Autodesk Fusion 360 part; units mm, degrees
sketch "スケッチ1" plane through (0, 0, 0) normal (0, 0, 1) x (1, 0, 0)
  line L0 (0, 0) -> (74, 0)
  line L1 (74, 0) -> (74, 46)
  line L2 (74, 46) -> (0, 46)
  line L3 (0, 46) -> (0, 0)
  dimension "d1" = 46
  dimension "d2" = 74
extrude "押し出し1" add sketch "スケッチ1" along normal blind 2
sketch "スケッチ2" plane through (0, 0, 2) normal (0, 0, 1) x (-1, 0, 0)
  line L0 (0, -46) -> (0, 0)
  line L1 (0, 0) -> (-74, 0)
  line L2 (-74, 0) -> (-74, -46)
  line L3 (-74, -46) -> (0, -46)
  line L4 (-27, -13) -> (-47, -13)
  line L5 (-47, -13) -> (-47, -15)
  line L6 (-47, -15) -> (-27, -15)
  line L7 (-27, -15) -> (-27, -13)
  dimension "d5" = 2
  dimension "d6" = 20
  dimension "d7" = 13
  dimension "d8" = 27
extrude "押し出し2" cut sketch "スケッチ2" against normal blind 2 contours L4 L5 L6 L7
sketch "スケッチ3" plane through (0, 0, 2) normal (0, 0, 1) x (-1, 0, 0)
  line L0 (-47, -13) -> (-27, -13)
  line L1 (-27, -13) -> (-27, -15)
  line L2 (-27, -15) -> (-47, -15)
  line L3 (-47, -15) -> (-47, -13)
  line L4 (0, -46) -> (0, 0)
  line L5 (0, 0) -> (-74, 0)
  line L6 (-74, 0) -> (-74, -46)
  line L7 (-74, -46) -> (0, -46)
  line L8 (-67, -46) -> (-58, -46)
  line L9 (-58, -46) -> (-58, -44)
  line L10 (-58, -44) -> (-67, -44)
  line L11 (-67, -44) -> (-67, -46)
  line L12 (-50, -46) -> (-41, -46)
  line L13 (-50, -44) -> (-50, -46)
  line L14 (-41, -44) -> (-50, -44)
  line L15 (-41, -46) -> (-41, -44)
  line L16 (-33, -46) -> (-24, -46)
  line L17 (-33, -44) -> (-33, -46)
  line L18 (-24, -44) -> (-33, -44)
  line L19 (-24, -46) -> (-24, -44)
  line L20 (-16, -46) -> (-7, -46)
  line L21 (-16, -44) -> (-16, -46)
  line L22 (-7, -44) -> (-16, -44)
  line L23 (-7, -46) -> (-7, -44)
  line L24 (-24, 0) -> (-33, 0)
  line L25 (-33, 0) -> (-33, -2)
  line L26 (-58, 0) -> (-67, 0)
  line L27 (-50, 0) -> (-50, -2)
  line L28 (-50, -2) -> (-41, -2)
  line L29 (-7, -2) -> (-7, 0)
  line L30 (-7, 0) -> (-16, 0)
  line L31 (-16, 0) -> (-16, -2)
  line L32 (-33, -2) -> (-24, -2)
  line L33 (-67, 0) -> (-67, -2)
  line L34 (-41, -2) -> (-41, 0)
  line L35 (-16, -2) -> (-7, -2)
  line L36 (-24, -2) -> (-24, 0)
  line L37 (-41, 0) -> (-50, 0)
  line L38 (-67, -2) -> (-58, -2)
  line L39 (-58, -2) -> (-58, 0)
  line L40 (0, -38) -> (-2, -38)
  line L41 (-2, -38) -> (-2, -32)
  line L42 (-2, -32) -> (0, -32)
  line L43 (0, -32) -> (0, -38)
  line L44 (-2, -20) -> (0, -20)
  line L45 (-2, -26) -> (-2, -20)
  line L46 (0, -26) -> (-2, -26)
  line L47 (0, -20) -> (0, -26)
  line L48 (-2, -8) -> (0, -8)
  line L49 (-2, -14) -> (-2, -8)
  line L50 (0, -14) -> (-2, -14)
  line L51 (0, -8) -> (0, -14)
  line L52 (-74, -20) -> (-72, -20)
  line L53 (-72, -8) -> (-72, -14)
  line L54 (-74, -8) -> (-72, -8)
  line L55 (-72, -14) -> (-74, -14)
  line L56 (-74, -38) -> (-74, -32)
  line L57 (-72, -32) -> (-72, -38)
  line L58 (-72, -26) -> (-74, -26)
  line L59 (-74, -32) -> (-72, -32)
  line L60 (-74, -14) -> (-74, -8)
  line L61 (-72, -20) -> (-72, -26)
  line L62 (-74, -26) -> (-74, -20)
  line L63 (-72, -38) -> (-74, -38)
  dimension "d11" = 9
  dimension "d12" = 2
  dimension "d13" = 7
  dimension "d16" = 17
  dimension "d17" = 0
  dimension "d20" = 0
  dimension "d21" = 44
  dimension "d22" = 6
  dimension "d23" = 2
  dimension "d24" = 8
  dimension "d27" = 0
  dimension "d28" = 12
  dimension "d31" = -72
  dimension "d32" = 0
extrude "押し出し3" cut sketch "スケッチ3" against normal blind 2 contours L4 L40 L41 L42 L43 | L7 L20 L21 L22 L23 | L4 L44 L45 L46 L47 | L7 L16 L17 L18 L19 | L4 L48 L49 L50 L51 | L7 L12 L13 L14 L15 | L7 L8 L9 L10 L11 | L5 L29 L30 L31 L35 | L5 L24 L25 L32 L36 | L6 L56 L57 L59 L63 | L5 L27 L28 L34 L37 | L6 L52 L58 L61 L62 | L5 L26 L33 L38 L39 | L6 L53 L54 L55 L60
sketch "スケッチ4" plane through (0, 0, 2) normal (0, 0, 1) x (-1, 0, 0)
  line L0 (-50, -2) -> (-50, 0)
  line L1 (-50, 0) -> (-58, 0)
  line L2 (-58, 0) -> (-58, -2)
  line L3 (-58, -2) -> (-67, -2)
  line L4 (-67, -2) -> (-67, 0)
  line L5 (-67, 0) -> (-74, 0)
  line L6 (-74, 0) -> (-74, -8)
  line L7 (-74, -8) -> (-72, -8)
  line L8 (-72, -8) -> (-72, -14)
  line L9 (-72, -14) -> (-74, -14)
  line L10 (-74, -14) -> (-74, -20)
  line L11 (-74, -20) -> (-72, -20)
  line L12 (-72, -20) -> (-72, -26)
  line L13 (-72, -26) -> (-74, -26)
  line L14 (-74, -26) -> (-74, -32)
  line L15 (-74, -32) -> (-72, -32)
  line L16 (-72, -32) -> (-72, -38)
  line L17 (-72, -38) -> (-74, -38)
  line L18 (-74, -38) -> (-74, -46)
  line L19 (-74, -46) -> (-67, -46)
  line L20 (-67, -46) -> (-67, -44)
  line L21 (-67, -44) -> (-58, -44)
  line L22 (-58, -44) -> (-58, -46)
  line L23 (-58, -46) -> (-50, -46)
  line L24 (-50, -46) -> (-50, -44)
  line L25 (-50, -44) -> (-41, -44)
  line L26 (-41, -44) -> (-41, -46)
  line L27 (-41, -46) -> (-33, -46)
  line L28 (-33, -46) -> (-33, -44)
  line L29 (-33, -44) -> (-24, -44)
  line L30 (-24, -44) -> (-24, -46)
  line L31 (-24, -46) -> (-16, -46)
  line L32 (-16, -46) -> (-16, -44)
  line L33 (-16, -44) -> (-7, -44)
  line L34 (-7, -44) -> (-7, -46)
  line L35 (-7, -46) -> (0, -46)
  line L36 (0, -46) -> (0, -38)
  line L37 (0, -38) -> (-2, -38)
  line L38 (-2, -38) -> (-2, -32)
  line L39 (-2, -32) -> (0, -32)
  line L40 (0, -32) -> (0, -26)
  line L41 (0, -26) -> (-2, -26)
  line L42 (-2, -26) -> (-2, -20)
  line L43 (-2, -20) -> (0, -20)
  line L44 (0, -20) -> (0, -14)
  line L45 (0, -14) -> (-2, -14)
  line L46 (-2, -14) -> (-2, -8)
  line L47 (-2, -8) -> (0, -8)
  line L48 (0, -8) -> (0, 0)
  line L49 (0, 0) -> (-7, 0)
  line L50 (-7, 0) -> (-7, -2)
  line L51 (-7, -2) -> (-16, -2)
  line L52 (-16, -2) -> (-16, 0)
  line L53 (-16, 0) -> (-24, 0)
  line L54 (-24, 0) -> (-24, -2)
  line L55 (-24, -2) -> (-33, -2)
  line L56 (-33, -2) -> (-33, 0)
  line L57 (-33, 0) -> (-41, 0)
  line L58 (-41, 0) -> (-41, -2)
  line L59 (-41, -2) -> (-50, -2)
  line L60 (-47, -13) -> (-27, -13)
  line L61 (-27, -13) -> (-27, -15)
  line L62 (-27, -15) -> (-47, -15)
  line L63 (-47, -15) -> (-47, -13)
  line L64 (0, 0) -> (0, 20)
  line L65 (0, 20) -> (-7, 20)
  line L66 (-7, 20) -> (-7, 0)
  line L67 (-74, 0) -> (-74, 20)
  line L68 (-74, 20) -> (-67, 20)
  line L69 (-67, 20) -> (-67, 0)
extrude "押し出し4" add sketch "スケッチ4" against normal blind 2 contours L5 L67 L68 L69 | L49 L64 L65 L66
sketch "スケッチ5" plane through (0, 0, 2) normal (0, 0, 1) x (-1, 0, 0)
  line L0 (-50, -2) -> (-50, 0)
  line L1 (-50, 0) -> (-58, 0)
  line L2 (-58, 0) -> (-58, -2)
  line L3 (-58, -2) -> (-67, -2)
  line L4 (-67, -2) -> (-67, 20)
  line L5 (-67, 20) -> (-74, 20)
  line L6 (-74, 20) -> (-74, -8)
  line L7 (-74, -8) -> (-72, -8)
  line L8 (-72, -8) -> (-72, -14)
  line L9 (-72, -14) -> (-74, -14)
  line L10 (-74, -14) -> (-74, -20)
  line L11 (-74, -20) -> (-72, -20)
  line L12 (-72, -20) -> (-72, -26)
  line L13 (-72, -26) -> (-74, -26)
  line L14 (-74, -26) -> (-74, -32)
  line L15 (-74, -32) -> (-72, -32)
  line L16 (-72, -32) -> (-72, -38)
  line L17 (-72, -38) -> (-74, -38)
  line L18 (-74, -38) -> (-74, -46)
  line L19 (-74, -46) -> (-67, -46)
  line L20 (-67, -46) -> (-67, -44)
  line L21 (-67, -44) -> (-58, -44)
  line L22 (-58, -44) -> (-58, -46)
  line L23 (-58, -46) -> (-50, -46)
  line L24 (-50, -46) -> (-50, -44)
  line L25 (-50, -44) -> (-41, -44)
  line L26 (-41, -44) -> (-41, -46)
  line L27 (-41, -46) -> (-33, -46)
  line L28 (-33, -46) -> (-33, -44)
  line L29 (-33, -44) -> (-24, -44)
  line L30 (-24, -44) -> (-24, -46)
  line L31 (-24, -46) -> (-16, -46)
  line L32 (-16, -46) -> (-16, -44)
  line L33 (-16, -44) -> (-7, -44)
  line L34 (-7, -44) -> (-7, -46)
  line L35 (-7, -46) -> (0, -46)
  line L36 (0, -46) -> (0, -38)
  line L37 (0, -38) -> (-2, -38)
  line L38 (-2, -38) -> (-2, -32)
  line L39 (-2, -32) -> (0, -32)
  line L40 (0, -32) -> (0, -26)
  line L41 (0, -26) -> (-2, -26)
  line L42 (-2, -26) -> (-2, -20)
  line L43 (-2, -20) -> (0, -20)
  line L44 (0, -20) -> (0, -14)
  line L45 (0, -14) -> (-2, -14)
  line L46 (-2, -14) -> (-2, -8)
  line L47 (-2, -8) -> (0, -8)
  line L48 (0, -8) -> (0, 20)
  line L49 (0, 20) -> (-7, 20)
  line L50 (-7, 20) -> (-7, -2)
  line L51 (-7, -2) -> (-16, -2)
  line L52 (-16, -2) -> (-16, 0)
  line L53 (-16, 0) -> (-24, 0)
  line L54 (-24, 0) -> (-24, -2)
  line L55 (-24, -2) -> (-33, -2)
  line L56 (-33, -2) -> (-33, 0)
  line L57 (-33, 0) -> (-41, 0)
  line L58 (-41, 0) -> (-41, -2)
  line L59 (-41, -2) -> (-50, -2)
  line L60 (-47, -13) -> (-27, -13)
  line L61 (-27, -13) -> (-27, -15)
  line L62 (-27, -15) -> (-47, -15)
  line L63 (-47, -15) -> (-47, -13)
  line L64 (0, -47) -> (-7, -47)
  line L65 (-7, -47) -> (-7, -46)
  line L66 (-7, -46) -> (0, -46)
  line L67 (0, -46) -> (0, -47)
  line L68 (-16, -46) -> (-24, -46)
  line L69 (-24, -46) -> (-24, -47)
  line L70 (-24, -47) -> (-16, -47)
  line L71 (-16, -47) -> (-16, -46)
  line L72 (-33, -46) -> (-41, -46)
  line L73 (-41, -46) -> (-41, -47)
  line L74 (-41, -47) -> (-33, -47)
  line L75 (-33, -47) -> (-33, -46)
  line L76 (-50, -46) -> (-58, -46)
  line L77 (-58, -46) -> (-58, -47)
  line L78 (-58, -47) -> (-50, -47)
  line L79 (-50, -47) -> (-50, -46)
  line L80 (-67, -46) -> (-75, -46)
  line L81 (-75, -46) -> (-75, -47)
  line L82 (-75, -47) -> (-67, -47)
  line L83 (-67, -47) -> (-67, -46)
  line L84 (-75, -46) -> (-74, -46)
  line L85 (-74, -46) -> (-74, -38)
  line L86 (-74, -38) -> (-75, -38)
  line L87 (-75, -38) -> (-75, -46)
  line L88 (-75, -32) -> (-74, -32)
  line L89 (-74, -32) -> (-74, -26)
  line L90 (-74, -26) -> (-75, -26)
  line L91 (-75, -26) -> (-75, -32)
  line L92 (-75, -20) -> (-74, -20)
  line L93 (-74, -20) -> (-74, -14)
  line L94 (-74, -14) -> (-75, -14)
  line L95 (-75, -14) -> (-75, -20)
  line L96 (-75, -8) -> (-74, -8)
  line L97 (-74, -8) -> (-74, 20)
  line L98 (-74, 20) -> (-75, 20)
  line L99 (-75, 20) -> (-75, -8)
  line L100 (-75, 21) -> (-67, 21)
  line L101 (-67, 21) -> (-67, 20)
  line L102 (-67, 20) -> (-75, 20)
  line L103 (-75, 20) -> (-75, 21)
  line L104 (-58, 0) -> (-50, 0)
  line L105 (-50, 0) -> (-50, 1)
  line L106 (-50, 1) -> (-58, 1)
  line L107 (-58, 1) -> (-58, 0)
  line L108 (-41, 0) -> (-33, 0)
  line L109 (-33, 0) -> (-33, 1)
  line L110 (-33, 1) -> (-41, 1)
  line L111 (-41, 1) -> (-41, 0)
  line L112 (-24, 0) -> (-16, 0)
  line L113 (-16, 0) -> (-16, 1)
  line L114 (-16, 1) -> (-24, 1)
  line L115 (-24, 1) -> (-24, 0)
  line L116 (-7, 20) -> (1, 20)
  line L117 (1, 20) -> (1, 21)
  line L118 (1, 21) -> (-7, 21)
  line L119 (-7, 21) -> (-7, 20)
  line L120 (1, 20) -> (0, 20)
  line L121 (0, 20) -> (0, -8)
  line L122 (0, -8) -> (1, -8)
  line L123 (1, -8) -> (1, 20)
  line L124 (1, -14) -> (0, -14)
  line L125 (0, -14) -> (0, -20)
  line L126 (0, -20) -> (1, -20)
  line L127 (1, -20) -> (1, -14)
  line L128 (1, -26) -> (0, -26)
  line L129 (0, -26) -> (0, -32)
  line L130 (0, -32) -> (1, -32)
  line L131 (1, -32) -> (1, -26)
  line L132 (0, -38) -> (1, -38)
  line L133 (1, -38) -> (1, -47)
  line L134 (1, -47) -> (0, -47)
  line L135 (0, -47) -> (0, -38)
extrude "押し出し5" add sketch "スケッチ5" against normal blind 2 contours L1 L104 L105 L106 L107 | L57 L108 L109 L110 L111 | L5 L98 L100 L101 L102 L103 | L6 L96 L97 L98 L99 L102 | L53 L112 L113 L114 L115 | L10 L92 L93 L94 L95 | L49 L116 L117 L118 L119 L120 | L48 L116 L120 L121 L122 L123 | L14 L88 L89 L90 L91 | L44 L124 L125 L126 L127 | L18 L80 L84 L85 L86 L87 | L19 L80 L81 L82 L83 L84 | L40 L128 L129 L130 L131 | L23 L76 L77 L78 L79 | L36 L67 L132 L133 L134 L135 | L35 L64 L65 L66 L67 L135 | L27 L72 L73 L74 L75 | L31 L68 L69 L70 L71
sketch "スケッチ6" plane through (0, 0, 2) normal (0, 0, 1) x (-1, 0, 0)
  line L0 (-50, -2) -> (-50, 1)
  line L1 (-50, 1) -> (-58, 1)
  line L2 (-58, 1) -> (-58, -2)
  line L3 (-58, -2) -> (-67, -2)
  line L4 (-67, -2) -> (-67, 21)
  line L5 (-67, 21) -> (-75, 21)
  line L6 (-75, 21) -> (-75, -8)
  line L7 (-75, -8) -> (-72, -8)
  line L8 (-72, -8) -> (-72, -14)
  line L9 (-72, -14) -> (-75, -14)
  line L10 (-75, -14) -> (-75, -20)
  line L11 (-75, -20) -> (-72, -20)
  line L12 (-72, -20) -> (-72, -26)
  line L13 (-72, -26) -> (-75, -26)
  line L14 (-75, -26) -> (-75, -32)
  line L15 (-75, -32) -> (-72, -32)
  line L16 (-72, -32) -> (-72, -38)
  line L17 (-72, -38) -> (-75, -38)
  line L18 (-75, -38) -> (-75, -47)
  line L19 (-75, -47) -> (-67, -47)
  line L20 (-67, -47) -> (-67, -44)
  line L21 (-67, -44) -> (-58, -44)
  line L22 (-58, -44) -> (-58, -47)
  line L23 (-58, -47) -> (-50, -47)
  line L24 (-50, -47) -> (-50, -44)
  line L25 (-50, -44) -> (-41, -44)
  line L26 (-41, -44) -> (-41, -47)
  line L27 (-41, -47) -> (-33, -47)
  line L28 (-33, -47) -> (-33, -44)
  line L29 (-33, -44) -> (-24, -44)
  line L30 (-24, -44) -> (-24, -47)
  line L31 (-24, -47) -> (-16, -47)
  line L32 (-16, -47) -> (-16, -44)
  line L33 (-16, -44) -> (-7, -44)
  line L34 (-7, -44) -> (-7, -47)
  line L35 (-7, -47) -> (1, -47)
  line L36 (1, -47) -> (1, -38)
  line L37 (1, -38) -> (-2, -38)
  line L38 (-2, -38) -> (-2, -32)
  line L39 (-2, -32) -> (1, -32)
  line L40 (1, -32) -> (1, -26)
  line L41 (1, -26) -> (-2, -26)
  line L42 (-2, -26) -> (-2, -20)
  line L43 (-2, -20) -> (1, -20)
  line L44 (1, -20) -> (1, -14)
  line L45 (1, -14) -> (-2, -14)
  line L46 (-2, -14) -> (-2, -8)
  line L47 (-2, -8) -> (1, -8)
  line L48 (1, -8) -> (1, 21)
  line L49 (1, 21) -> (-7, 21)
  line L50 (-7, 21) -> (-7, -2)
  line L51 (-7, -2) -> (-16, -2)
  line L52 (-16, -2) -> (-16, 1)
  line L53 (-16, 1) -> (-24, 1)
  line L54 (-24, 1) -> (-24, -2)
  line L55 (-24, -2) -> (-33, -2)
  line L56 (-33, -2) -> (-33, 1)
  line L57 (-33, 1) -> (-41, 1)
  line L58 (-41, 1) -> (-41, -2)
  line L59 (-41, -2) -> (-50, -2)
  line L60 (-47, -13) -> (-27, -13)
  line L61 (-27, -13) -> (-27, -15)
  line L62 (-27, -15) -> (-47, -15)
  line L63 (-47, -15) -> (-47, -13)
Geometry: final body of the model. Coordinates: model frame, mm. A direction names the side the tool comes from. Coordinates: 2 decimals unless noted, no trailing zeros. Loops run counter-clockwise (first coordinate to the right, second up) from the corner with the lowest first, then second, coordinate; pieces in that order, holes last. Notation, with made-up numbers: M 88.5,-3.75 L 107.5,-3.75 A17 ccw 107.5,23.25 Z; hole C 40.5,5.5 d7. An arc over 180 degrees is marked long. Put each result on its own line as item: value.
(1) Cut plane D-D on x = 61.5. Return the cut outline in (y, z).
Answer sheet:
outline: M 2,0 L 44,0 L 44,2 L 2,2 Z
(2) Draft query along Y for faces 1 (the face through (1, 8, 1)), 2 (the face through (67, -10, 1)), 3 (the face through (37, -1, 1)). Return one class per face: pulls with the +Y half, pulls with the -Y half, needs draft (parallel to the pull), parting line crosses it, or undercut.
Answer sheet:
face 1: undercut
face 2: needs draft
face 3: pulls with the -Y half
(3) Material intervals for probe 1 along Y at (x, z) = (36.5, 1.45); probe 2 along X at (y, z) = (44.5, 1.45); probe 3 along Y at (x, z) = (42, 0.3), sorted ascending.
Answer sheet:
probe 1: y = -1 to 13, 15 to 47
probe 2: x = -1 to 7, 16 to 24, 33 to 41, 50 to 58, 67 to 75
probe 3: y = 2 to 13, 15 to 44
(4) Access query for faces 4 (the face through (1, 32, 1)), 5 (the face through (47, 14, 1)), 6 (the face through (16, 45, 1)), 7 (the face through (72, 23, 1)). Directions: +Z, -Z, +X, -X, +Y, -Y. A direction counts if a zero-diameter tool reaches every point of the face in a straight line with its end or side. Return the directions, or none.
Answer sheet:
face 4: +Z, -Z, -X
face 5: +Z, -Z
face 6: +Z, -Z, +Y
face 7: +Z, -Z, +X
(5) Cut plane C-C on y = 11. Return the cut outline in (x, z), then the cut area to 3 significant figures.
Answer sheet:
outline: M 2,0 L 72,0 L 72,2 L 2,2 Z
area: 140 mm^2
(6) Cut plane A-A on x = 34.5. Return the cut outline in (y, z).
Answer sheet:
outline: M -1,0 L 13,0 L 13,2 L -1,2 Z; M 15,0 L 47,0 L 47,2 L 15,2 Z
(7) Cut plane B-B on y = -3. Return the cut outline in (x, z), then the cut area to 3 significant figures.
Answer sheet:
outline: M -1,0 L 7,0 L 7,2 L -1,2 Z; M 67,0 L 75,0 L 75,2 L 67,2 Z
area: 32.0 mm^2
(8) First-contact query: pin 1 (1 mm diameter, centred on x = 28, z = 1.5, fed in from -Y); pin 2 (10 mm diameter, centred on x = 61.5, y = 33.5, fed in from -Z); pin 3 (1 mm diameter, centred on x = 54.5, z = 1.5, fed in from -Y); pin 4 (1 mm diameter, centred on y = 12, z = 1.5, fed in from +X). Flat tips, straight axial feed; report the tip coordinate or a pass-through.
Answer sheet:
pin 1: stops at y = 2
pin 2: stops at z = 0
pin 3: stops at y = -1
pin 4: stops at x = 72
